from build123d import *

# Parameters (mm, degrees)
EXTRUDE1_DEPTH             = 250
SKETCH2_R                  = 1.75
EXTRUDE2_DEPTH             = 6.5
SKETCH_R                   = 3
SKETCH_R_2                 = 1.75
EXTRUDE4_DEPTH             = 3.5
CHAMFER1_SIZE              = 0.2
LPATTERN1_COUNT            = 12
LPATTERN1_PITCH            = 20
CHAMFER1_OF_LPATTERN1_SIZE = 0.2


with BuildPart() as part:
    # Sketch1 → Extrude1 (new body)
    with BuildSketch(Plane.XY):
        with BuildLine():
            Line((-4.3, -3.25), (4.3, -3.25))
            Line((4.3, -3.25), (4.5, -3.05))
            Line((4.5, -3.05), (4.5, 0.455012563))
            ThreePointArc((4.5, 0.455012563), (3.924845827, 0.712323349), (3.617735397, 1.2625))
            Line((3.617735397, 1.2625), (3.15008224, 1.2625))
            Line((3.15008224, 1.2625), (3.15008224, 1.7625))
            Line((3.15008224, 1.7625), (3.65008224, 1.7625))
            ThreePointArc((3.65008224, 1.7625), (3.973877727, 2.229724887), (4.5, 2.444987437))
            Line((4.5, 2.444987437), (4.5, 3.05))
            Line((4.5, 3.05), (4.3, 3.25))
            Line((4.3, 3.25), (-4.3, 3.25))
            Line((-4.3, 3.25), (-4.5, 3.05))
            Line((-4.5, 3.05), (-4.5, 2.444987437))
            ThreePointArc((-4.5, 2.444987437), (-3.973877727, 2.229724887), (-3.65008224, 1.7625))
            Line((-3.65008224, 1.7625), (-3.15008224, 1.7625))
            Line((-3.15008224, 1.7625), (-3.15008224, 1.2625))
            Line((-3.15008224, 1.2625), (-3.617735397, 1.2625))
            ThreePointArc((-3.617735397, 1.2625), (-3.924845827, 0.712323349), (-4.5, 0.455012563))
            Line((-4.5, 0.455012563), (-4.5, -3.05))
            Line((-4.5, -3.05), (-4.3, -3.25))
        make_face()
    extrude(amount=EXTRUDE1_DEPTH)

    # Sketch2 → Extrude2 (cut)
    with BuildSketch(Plane(origin=(0, 3.25, 0), x_dir=(1, 0, 0), z_dir=(0, 1, 0))):
        with Locations((0, -15)):
            Circle(SKETCH2_R)
    extrude2 = extrude(amount=-EXTRUDE2_DEPTH, mode=Mode.SUBTRACT)

    # Sketch → Extrude4 (cut)
    with BuildSketch(Plane(origin=(0, 3.25, 0), x_dir=(1, 0, 0), z_dir=(0, 1, 0))):
        with Locations((0, -15)):
            Circle(SKETCH_R)
        with Locations((0, -15)):
            Circle(SKETCH_R_2, mode=Mode.SUBTRACT)
    extrude4 = extrude(amount=-EXTRUDE4_DEPTH, mode=Mode.SUBTRACT)

    # Chamfer1
    chamfer1_edges = [part.edges().sort_by_distance(p)[0] for p in [
        (-1.75, -3.25, 15),
        (-3, 3.25, 15),
    ]]
    chamfer(chamfer1_edges, length=CHAMFER1_SIZE)

    # LPattern1: Extrude2, Extrude4 ×12
    with Locations(*[(0, 0, i * LPATTERN1_PITCH) for i in range(1, LPATTERN1_COUNT)]):
        add(extrude2, mode=Mode.SUBTRACT)
        add(extrude4, mode=Mode.SUBTRACT)

    # Chamfer1 of LPattern1
    chamfer1_of_lpattern1_edges = [part.edges().sort_by_distance(p)[0] for p in [
        (-1.75, -3.25, 35),
        (-3, 3.25, 35),
        (-1.75, -3.25, 55),
        (-3, 3.25, 55),
        (-1.75, -3.25, 75),
        (-3, 3.25, 75),
        (-1.75, -3.25, 95),
        (-3, 3.25, 95),
        (-1.75, -3.25, 115),
        (-3, 3.25, 115),
        (-1.75, -3.25, 135),
        (-3, 3.25, 135),
        (-1.75, -3.25, 155),
        (-3, 3.25, 155),
        (-1.75, -3.25, 175),
        (-3, 3.25, 175),
        (-1.75, -3.25, 195),
        (-3, 3.25, 195),
        (-1.75, -3.25, 215),
        (-3, 3.25, 215),
        (-1.75, -3.25, 235),
        (-3, 3.25, 235),
    ]]
    chamfer(chamfer1_of_lpattern1_edges, length=CHAMFER1_OF_LPATTERN1_SIZE)


solid = part.part
Verification items for the finished model (mm, model axes). Coordinates: 2 decimals unless noted, no trailing zeros. Order: outer loops, then holes, each group sorted by start corner. A loop starts at its lowest first (then second) coordinate and runs counter-clockwise, first axis right, second up. Notation, with made-up numbers: M 74.25,58 L 103.25,58 A27 ccw 103.25,88 Z; hole C 76,55.5 d10. An arc over 180 degrees is marked long. One line per item, written item: value. Start each with the question number.
Item 1: Mould release check, pull along Z, two halves, no side actions. Record for faces 1 (the flat face through (0, 0, 250)), 2 (the flat face through (2, -0.25, 175)), 3 (the flat face through (0, -0.25, 37)), 4 (the flat face through (0, -3.25, 123)): released by +Z, released by -Z, zero draft, split by the parting line, or undercut.
Item 2: Gauge pin test, flat ends, axial feed: pin 1 (4.5 mm diameter, centred on x = 0, z = 215, fed in from +Y); pin 2 (2 mm diameter, centred on x = 0, z = 35, fed in from +Y) (1 decimal). Record the tip position at first contact, or that the pin passes through.
Item 3: Sectioned sample at A-A (y = -1.5). Count the separate pieces of the cut face and the enclosed holes in it, then the cut area to 3 significant figures.
Item 4: Scan lines: probe 1 along X at (y, z) = (1.3, 55); probe 2 along Y at (x, z) = (3.75, 186); probe 3 along X at (y, z) = (-1.25, 134). Record each from-to range of solid material in increasing order.
Item 5: Sectioned sample at B-B (z = 83). Enter the section's corners in (x, y), then the cut area to 3 significant figures.
Conclusion:
1. face 1: released by +Z
1. face 2: undercut
1. face 3: undercut
1. face 4: zero draft
2. pin 1: stops at y = -0.25
2. pin 2: passes through
3. separate pieces: 1
3. enclosed holes: 12
3. area: 2,130 mm^2
4. probe 1: x = -3.15 to -3, 3 to 3.15
4. probe 2: y = -3.25 to 0.92, 1.98 to 3.25
4. probe 3: x = -4.5 to -1.44, 1.44 to 4.5
5. outline: M -4.5,-3.05 L -4.3,-3.25 L 4.3,-3.25 L 4.5,-3.05 L 4.5,0.46 A1 cw 3.62,1.26 L 3.15,1.26 L 3.15,1.76 L 3.65,1.76 A1 cw 4.5,2.44 L 4.5,3.05 L 4.3,3.25 L -4.3,3.25 L -4.5,3.05 L -4.5,2.44 A1 cw -3.65,1.76 L -3.15,1.76 L -3.15,1.26 L -3.62,1.26 A1 cw -4.5,0.46 Z
5. area: 55.2 mm^2
